Part model, mm, in its own coordinate system. A direction names the side the tool comes from. Coordinates: 2 decimals unless noted, no trailing zeros. Order: outer loops, then holes, each group sorted by start corner. A loop starts at its lowest first (then second) coordinate and runs counter-clockwise, first axis right, second up.
```python
from build123d import *

# Parameters (mm, degrees)
F1_DEPTH      = 60
F1_DEPTH_BACK = 1.2
F0_W          = 15
F0_H          = 7
F2_DEPTH      = 1.2


with BuildPart() as f1:
    # F0 (on Top) → F1 (new body, two sides)
    with BuildSketch(Plane.XY) as f1_sk:
        with BuildLine():
            Line((-12.45, 7.5), (-12.45, -7.5))
            ThreePointArc((-12.45, -7.5), (-11.952082, -8.702082), (-10.75, -9.2))
            Line((-10.75, -9.2), (10.75, -9.2))
            ThreePointArc((10.75, -9.2), (11.952082, -8.702082), (12.45, -7.5))
            Line((12.45, -7.5), (12.45, 7.5))
            ThreePointArc((12.45, 7.5), (11.952082, 8.702082), (10.75, 9.2))
            Line((10.75, 9.2), (-10.75, 9.2))
            ThreePointArc((-10.75, 9.2), (-11.952082, 8.702082), (-12.45, 7.5))
        make_face()
        with BuildLine():
            ThreePointArc((11.25, -7.5), (11.103553, -7.853553), (10.75, -8))
            Line((10.75, -8), (-10.75, -8))
            ThreePointArc((-10.75, -8), (-11.103553, -7.853553), (-11.25, -7.5))
            Line((-11.25, -7.5), (-11.25, 7.5))
            ThreePointArc((-11.25, 7.5), (-11.103553, 7.853553), (-10.75, 8))
            Line((-10.75, 8), (10.75, 8))
            ThreePointArc((10.75, 8), (11.103553, 7.853553), (11.25, 7.5))
            Line((11.25, 7.5), (11.25, -7.5))
        make_face(mode=Mode.SUBTRACT)
    extrude(amount=F1_DEPTH)
    extrude(f1_sk.sketch, amount=-F1_DEPTH_BACK)

    # F0 (on Top) → F2 (join)
    with BuildSketch(Plane.XY):
        with BuildLine():
            Line((-10.75, -8), (10.75, -8))
            ThreePointArc((10.75, -8), (11.103553, -7.853553), (11.25, -7.5))
            Line((11.25, -7.5), (11.25, 7.5))
            ThreePointArc((11.25, 7.5), (11.103553, 7.853553), (10.75, 8))
            Line((10.75, 8), (-10.75, 8))
            ThreePointArc((-10.75, 8), (-11.103553, 7.853553), (-11.25, 7.5))
            Line((-11.25, 7.5), (-11.25, -7.5))
            ThreePointArc((-11.25, -7.5), (-11.103553, -7.853553), (-10.75, -8))
        make_face()
        with Locations((0, -1.5)):
            Rectangle(F0_W, F0_H, mode=Mode.SUBTRACT)
    extrude(amount=-F2_DEPTH)


solid = f1.part
```
(1) Pull direction X, two halves, no side cores. Call faces 4 (the face through (7.5, -2, -1)), 5 (the face through (-0.1, 8.2, 60)), 6 (the face through (0, 2, -1)), 7 (the face through (-11.965, -8.689, 29.828)): +X half, -X half, draft (parallel to the pull), parting line (faces both ways), or undercut.
(2) Tool access for faces 1 (the face through (-12.45, 0, 30)), 2 (the face through (0, 4, 0)), 3 (the face through (-7.5, -2, -1)): list every direction of +Z, -Z, +X, -X, +Y, -Y with a clear straight run to the whole face (end or side of a thin tool).
(3) Slice it at D-D, the plane x = 8.25. Give the cut face in (y, z), then the cut area to 3 significant figures.
(4) Slice it at A-A, the plane z = 17. Give the cut face in (x, y), then the cut area to 3 significant figures.
(5) Probe line 1 (Y direction, x = 2.25, z = 39); line 2 (X direction, y = -0.5, z = 48.5); line 3 (Z direction, x = 9.5, y = -0.25). List the from-to ranges inside material, lowest first.
(6) Slice it at B-B, the plane x = 1.75. Give the cut face in (y, z), then the cut area to 3 significant figures.
(7) Slice it at C-C, the plane y = -2.25. Give the cut face in (x, z), then the cut area to 3 significant figures.
(8) Drop a flat-ended pin along its axis: pin 1 (8 mm diameter, centred on x = 3.5, y = -0.5, fed in from +Z). Give the stop position or say it passes through.
Here are the results:
1. face 4: undercut
1. face 5: draft
1. face 6: undercut
1. face 7: -X half
2. face 1: +Z, -Z, -X, +Y, -Y
2. face 2: +Z
2. face 3: +Z, -Z
3. outline: (-9.2, -1.2) - (9.2, -1.2) - (9.2, 60) - (8, 60) - (8, 0) - (-8, 0) - (-8, 60) - (-9.2, 60) - close
3. area: 166 mm2
4. outline: (-12.45, -7.5) arc R1.7 ccw to (-10.75, -9.2) - (10.75, -9.2) arc R1.7 ccw to (12.45, -7.5) - (12.45, 7.5) arc R1.7 ccw to (10.75, 9.2) - (-10.75, 9.2) arc R1.7 ccw to (-12.45, 7.5) - close; hole (-11.25, -7.5) arc R0.5 ccw to (-10.75, -8) - (10.75, -8) arc R0.5 ccw to (11.25, -7.5) - (11.25, 7.5) arc R0.5 ccw to (10.75, 8) - (-10.75, 8) arc R0.5 ccw to (-11.25, 7.5) - close
4. area: 95.9 mm2
5. line 1: y = -9.2 to -8, 8 to 9.2
5. line 2: x = -12.45 to -11.25, 11.25 to 12.45
5. line 3: z = -1.2 to 0
6. outline: (-9.2, -1.2) - (-5, -1.2) - (-5, 0) - (-8, 0) - (-8, 60) - (-9.2, 60) - close; (2, -1.2) - (9.2, -1.2) - (9.2, 60) - (8, 60) - (8, 0) - (2, 0) - close
6. area: 158 mm2
7. outline: (-12.45, -1.2) - (-7.5, -1.2) - (-7.5, 0) - (-11.25, 0) - (-11.25, 60) - (-12.45, 60) - close; (7.5, -1.2) - (12.45, -1.2) - (12.45, 60) - (11.25, 60) - (11.25, 0) - (7.5, 0) - close
7. area: 156 mm2
8. pin 1: stops at z = 0
